from build123d import *

# Parameters (mm, degrees)
SKETCH1_R           = 31.75
BOSS_EXTRUDE1_DEPTH = 6.35
CHAMFER2_SIZE       = 2.54
SKETCH2_R           = 9.525
SKETCH2_R_2         = 1.5875
BOSS_EXTRUDE2_DEPTH = 2.54
SKETCH2_2_R         = 1.5875
CUT_EXTRUDE1_DEPTH  = 46.348070521
FILLET1_R           = 2.286
CUT_EXTRUDE4_DEPTH  = 46.772886079
CIRPATTERN1_COUNT   = 9
SKETCH5_W           = 24.13
SKETCH5_H           = 3.81
CUT_EXTRUDE5_DEPTH  = 1.524


with BuildPart() as part:
    # Sketch1 → Boss-Extrude1 (new body)
    with BuildSketch(Plane(origin=(0, 0, 0), x_dir=(1, 0, 0), z_dir=(0, 1, 0))):
        with Locations(Location((0, 0, 0), (0, 0, 270))):
            Circle(SKETCH1_R)
    extrude(amount=BOSS_EXTRUDE1_DEPTH)

    # Chamfer2
    chamfer2_edges = [part.edges().sort_by_distance(p)[0] for p in [
        (0, 6.35, -31.75),
    ]]
    chamfer(chamfer2_edges, length=CHAMFER2_SIZE)

    # Sketch2 → Boss-Extrude2 (add)
    with BuildSketch(Plane(origin=(0, 6.35, 0), x_dir=(1, 0, 0), z_dir=(0, 1, 0))):
        with Locations(Location((0, 15.875, 0), (0, 0, 270))):
            Circle(SKETCH2_R)
        with Locations(Location((0, 15.875, 0), (0, 0, 270))):
            Circle(SKETCH2_R_2, mode=Mode.SUBTRACT)
    extrude(amount=BOSS_EXTRUDE2_DEPTH)

    # Sketch2_2 → Cut-Extrude1 (cut, through all)
    with BuildSketch(Plane(origin=(0, 6.35, 0), x_dir=(1, 0, 0), z_dir=(0, 1, 0))):
        with Locations(Location((0, 15.875, 0), (0, 0, 270))):
            Circle(SKETCH2_2_R)
    extrude(amount=-CUT_EXTRUDE1_DEPTH, mode=Mode.SUBTRACT)

    # Fillet1
    fillet1_edges = [part.edges().sort_by_distance(p)[0] for p in [
        (0, 8.89, -25.4),
    ]]
    fillet(fillet1_edges, radius=FILLET1_R)

    # Sketch4 → Cut-Extrude4 (cut, through all)
    with BuildSketch(Plane(origin=(0, 8.89, 0), x_dir=(1, 0, 0), z_dir=(0, 1, 0))):
        with BuildLine():
            Line((9.503809762, 16.51), (6.963809762, 16.51))
            Line((6.963809762, 16.51), (6.963809762, 15.24))
            Line((6.963809762, 15.24), (9.503809762, 15.24))
            ThreePointArc((9.503809762, 15.24), (9.525, 15.875), (9.503809762, 16.51))
        make_face()
    cut_extrude4 = extrude(amount=-CUT_EXTRUDE4_DEPTH, mode=Mode.SUBTRACT)

    # CirPattern1: Cut-Extrude4 ×9 about axis
    cirpattern1_axis = Axis((0, 0, -15.875), (0, 1, 0))
    for i in range(1, CIRPATTERN1_COUNT):
        add(cut_extrude4.rotate(cirpattern1_axis, i * 360 / CIRPATTERN1_COUNT), mode=Mode.SUBTRACT)

    # Sketch5 → Cut-Extrude5 (cut)
    with BuildSketch(Plane(origin=(0, 6.35, 0), x_dir=(1, 0, 0), z_dir=(0, 1, 0))):
        with Locations((-18.3554105, 0)):
            Rectangle(SKETCH5_W, SKETCH5_H)
        with BuildLine():
            Line((-6.2904105, -3.175), (-6.2904105, -6.985))
            Line((-6.2904105, -6.985), (-29.668841821, -6.985))
            ThreePointArc((-29.668841821, -6.985), (-30.053265488, -5.090106258), (-30.319295317, -3.175))
            Line((-30.319295317, -3.175), (-6.2904105, -3.175))
        make_face()
        with BuildLine():
            Line((-6.2904105, -13.493377405), (-6.2904105, -9.683377405))
            Line((-6.2904105, -9.683377405), (-28.900910055, -9.683377405))
            ThreePointArc((-28.900910055, -9.683377405), (-28.18019525, -11.614947079), (-27.330553712, -13.493377405))
            Line((-27.330553712, -13.493377405), (-6.2904105, -13.493377405))
        make_face()
        with BuildLine():
            Line((-6.2904105, -16.033377405), (-6.2904105, -19.843377405))
            Line((-6.2904105, -19.843377405), (-23.135919544, -19.843377405))
            ThreePointArc((-23.135919544, -19.843377405), (-24.602929827, -17.992394058), (-25.922214585, -16.033377405))
            Line((-25.922214585, -16.033377405), (-6.2904105, -16.033377405))
        make_face()
    extrude(amount=-CUT_EXTRUDE5_DEPTH, mode=Mode.SUBTRACT)

    # Sketch6 → Cut-Revolve1 (revolve, cut)
    with BuildSketch(Plane(origin=(0, 0, 0), x_dir=(0, 0, -1), z_dir=(1, 0, 0)), mode=Mode.PRIVATE) as cut_revolve1_sk:
        Polygon((-30.48, 3.283948776), (-28.683948776, 5.08), (0, 5.08), (0, -0.561099899), (-30.990180808, -0.561099899), (-30.990180808, 1.27), (-30.48, 1.27), align=None)
    revolve(cut_revolve1_sk.sketch.rotate(Axis((0, 0, 0), (0, -1, 0)), 93.739333894), axis=Axis((0, 0, 0), (0, -1, 0)), mode=Mode.SUBTRACT)


solid = part.part
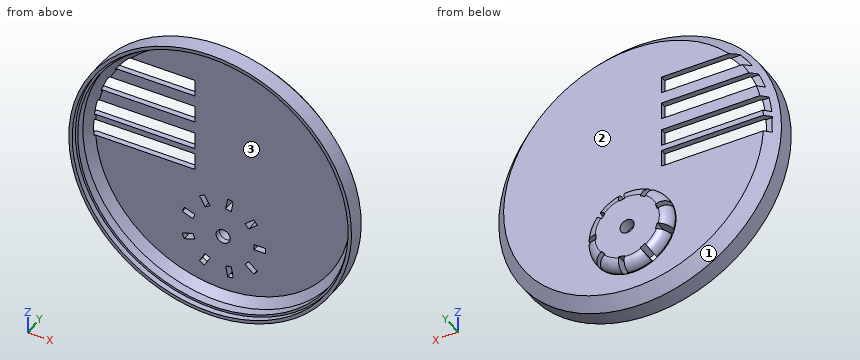
Geometry: final body of the model. Coordinates: model frame, mm. Face numbers are marked on the shaded views. Round coordinates to 2 decimals unless told otherwise and drop trailing zeros. Loops run counter-clockwise (first coordinate to the right, second up) from the corner with the lowest first, then second, coordinate; pieces in that order, holes last.
Q1. Pin query (flat end, axial travel): P1, Ø3, axis at x = 13, y = 6, coming from the +Z side; P2, Ø3, axis at x = 13.5, z = 0.5, coming from the +Y side; P3, Ø1, axis at y = 5.5, z = 11.5, coming from the -X side. Return the tip coordinate at first contact, or that it passes through.
Q2. Material intervals for L1, parallel to X at y = 2.15, z = 0; L2, parallel to Z at x = -4, y = 6.5; L3, parallel to Y at x = -22, z = -4.5, sorted ascending.
Q3. Section B-B on x = -18. State how many separate pieces and enclosed holes the cut face has, plus the area to 3 significant figures.
Q4. Section A-A on z = 0. Return loops of the section in (x, y), plus the area to 3 significant figures.
Q5. Pull-direction query (X, two-part tool) for the marked faces 1, 2 and 3; classes: released by +X, released by -X, zero draft, split by the parting line, or undercut.
Evaluation:
1. P1: stops at z = 28.34
1. P2: stops at y = 6.35
1. P3: stops at x = -28.35
2. L1: x = -31.75 to -30.48, 30.48 to 31.75
2. L2: z = -24.52 to -24.07, -21.61 to -10.14, -7.68 to -7.23
2. L3: y = 5.08 to 6.35
3. separate pieces: 5
3. enclosed holes: 0
3. area: 57.4 mm2
4. outline: (-31.75, 0) - (-30.99, 0) - (-30.99, 1.27) - (-30.48, 1.27) - (-30.48, 3.28) - (-28.94, 4.83) - (-30.42, 4.83) - (-30.42, 5.14) - (-31.75, 3.81) - close; (-6.29, 5.08) - (28.68, 5.08) - (30.48, 3.28) - (30.48, 1.27) - (30.99, 1.27) - (30.99, 0) - (31.75, 0) - (31.75, 3.81) - (29.21, 6.35) - (-6.29, 6.35) - close
4. area: 58.7 mm2
5. face 1: split by the parting line
5. face 2: zero draft
5. face 3: undercut
